from build123d import *

# Parameters (mm, degrees)
SKETCH1_W           = 25.4
SKETCH1_H           = 25.4
SKETCH1_W_2         = 19.05
SKETCH1_H_2         = 19.05
BOSS_EXTRUDE1_DEPTH = 381
SKETCH2_R           = 2.5
CUT_EXTRUDE1_DEPTH  = 26.4
SKETCH3_R           = 4.539166488
CUT_EXTRUDE2_DEPTH  = 26.4


with BuildPart() as part:
    # Sketch1 → Boss-Extrude1 (new body)
    with BuildSketch(Plane(origin=(0, 0, 0), x_dir=(1, 0, 0), z_dir=(0, 1, 0))):
        Rectangle(SKETCH1_W, SKETCH1_H)
        Rectangle(SKETCH1_W_2, SKETCH1_H_2, mode=Mode.SUBTRACT)
    extrude(amount=BOSS_EXTRUDE1_DEPTH)

    # Sketch2 → Cut-Extrude1 (cut, through all)
    with BuildSketch(Plane(origin=(0, 0, -12.7), x_dir=(-1, 0, 0), z_dir=(0, 0, -1))):
        with Locations((0, 20)):
            Circle(SKETCH2_R)
    extrude(amount=-CUT_EXTRUDE1_DEPTH, mode=Mode.SUBTRACT)

    # Sketch3 → Cut-Extrude2 (cut, through all)
    with BuildSketch(Plane.ZY.offset(12.7)):
        with Locations((0, 348.5)):
            Circle(SKETCH3_R)
        with Locations((0, 323.5)):
            Circle(SKETCH3_R)
    extrude(amount=-CUT_EXTRUDE2_DEPTH, mode=Mode.SUBTRACT)


solid = part.part
The model under review builds one solid part; all positions refer to its coordinate system, in mm. A direction names the side the tool comes from. Round coordinates to 2 decimals unless told otherwise and drop trailing zeros. Loops run counter-clockwise (first coordinate to the right, second up) from the corner with the lowest first, then second, coordinate; pieces in that order, holes last. Notation, with made-up numbers: (28.25, 82) - (36.25, 82) arc R26 cw to (36.25, 118) - close; hole circle Ø7 at (-13, 62). An arc over 180 degrees is marked (long way). Use CSV: the item, a comma, the result in double quotes.
(1) Machinability: for faces 1 (the flat face through (-12.7, 188, 0)), 2 (the flat face through (0, 188, -9.525)), which of the approach directions +Z, -Z, +X, -X, +Y, -Y give a long, thin tool a straight path to every point of the face, cutting with its end or side? Answer none if there is none.
Working result:
face 1,"+Z, -Z, -X, +Y, -Y"
face 2,"+Y, -Y"
(2) For line 1 (Y direction, x = 10.55, z = 0); line 2 (X direction, y = 231, z = 3) (3 decimals); line 3 (Y direction, x = 0, z = -11.6), list the stretches that pass through material, from the lowest coordinate up.
Working result:
line 1,"y = 0 to 318.96, 328.04 to 343.96, 353.04 to 381"
line 2,"x = -12.7 to -9.525, 9.525 to 12.7"
line 3,"y = 0 to 17.5, 22.5 to 381"
(3) Clearance check with a flat-ended pin moving along its axis: P1, Ø7.5, axis at y = 323.5, z = 0, coming from the +X side. State where the tip first meets the part, or that it passes through.
Working result:
P1,"passes through"
(4) Take a section at B-B, the plane y = 222. Give the boundary of the cut face in (x, z) (3 decimals).
Working result:
outline,"(-12.7, -12.7) - (12.7, -12.7) - (12.7, 12.7) - (-12.7, 12.7) - close; hole (-9.525, -9.525) - (9.525, -9.525) - (9.525, 9.525) - (-9.525, 9.525) - close"
(5) The part is to be moulded in two halves that separate along Z. For faces 3 (the flat face through (12.7, 188, 0)), 4 (the flat face through (0, 188, -12.7)), 5 (the cylindrical face through (-11.135, 344.069, -0.984)), 6 (the cylindrical face through (-11.135, 319.069, -0.984)), say which applies: pulls with the +Z half, pulls with the -Z half, needs draft (parallel to the pull), parting line crosses it, or undercut.
Working result:
face 3,"needs draft"
face 4,"pulls with the -Z half"
face 5,"undercut"
face 6,"undercut"
(6) Take a section at A-A, the plane y = 348.5. Give the boundary of the cut face in (x, z) (3 decimals).
Working result:
outline,"(-12.7, -12.7) - (12.7, -12.7) - (12.7, -4.539) - (9.525, -4.539) - (9.525, -9.525) - (-9.525, -9.525) - (-9.525, -4.539) - (-12.7, -4.539) - close; (-12.7, 4.539) - (-9.525, 4.539) - (-9.525, 9.525) - (9.525, 9.525) - (9.525, 4.539) - (12.7, 4.539) - (12.7, 12.7) - (-12.7, 12.7) - close"
